The model under review builds one solid part; all positions refer to its coordinate system, in mm. Face numbers are marked on the shaded views. A direction names the side the tool comes from. Coordinates: 2 decimals unless noted, no trailing zeros. Loops run counter-clockwise (first coordinate to the right, second up) from the corner with the lowest first, then second, coordinate; pieces in that order, holes last. Notation, with made-up numbers: M -29.5,-27.75 L -11.5,-27.75 A12 cw -11.5,-18.75 Z; hole C 72.5,40 d7. An arc over 180 degrees is marked long. Use one line per item in the form item = value.
```python
from build123d import *

# Parameters (mm, degrees)
F0_W     = 22
F0_H     = 22
F0_W_2   = 14
F0_H_2   = 14
F1_DEPTH = 1.45
F2_W     = 22
F2_H     = 22
F2_W_2   = 15
F2_H_2   = 15
F3_DEPTH = 7
F4_SIZE  = 3


with BuildPart() as f1:
    # F0 (on Front) → F1 (new body)
    with BuildSketch(Plane.XZ):
        Rectangle(F0_W, F0_H)
        Rectangle(F0_W_2, F0_H_2, mode=Mode.SUBTRACT)
    extrude(amount=F1_DEPTH)

    # F2 (on face) → F3 (join)
    with BuildSketch(Plane.XZ.offset(1.45)):
        Rectangle(F2_W, F2_H)
        Rectangle(F2_W_2, F2_H_2, mode=Mode.SUBTRACT)
    extrude(amount=F3_DEPTH)

    # F4
    f4_edges = [f1.edges().sort_by_distance(p)[0] for p in [
        (-11, -4.225, 11),
        (11, -4.225, 11),
        (11, -4.225, -11),
        (-11, -4.225, -11),
    ]]
    chamfer(f4_edges, length=F4_SIZE)


solid = f1.part
```
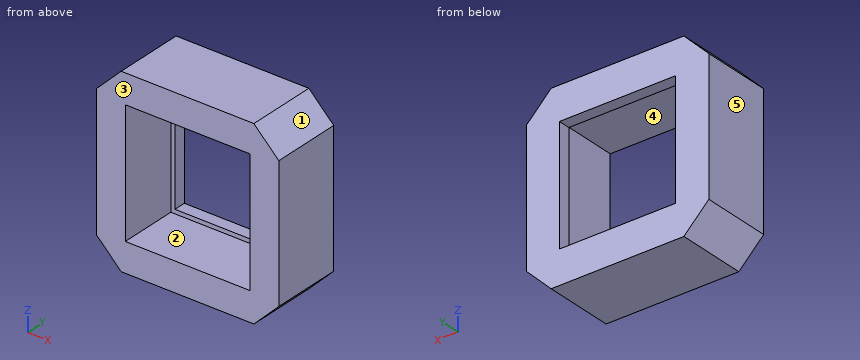
1. Machinability: for the marked faces 4 and 5, which of the approach directions +Z, -Z, +X, -X, +Y, -Y give a long, thin tool a straight path to every point of the face, cutting with its end or side? Answer none if there is none.
Response values:
face_4 = -Y
face_5 = +Z, -Z, -X, +Y, -Y
2. Wall thickness on line 1 along Z through (x, y) = (-6, -4); line 2 along X through (y, z) = (-1, -5.25): over which ranges is each line inside the solid? List them lowest first. Write a range as from..to.
Response values:
line_1 = -11..-7.5, 7.5..11
line_2 = -11..-7, 7..11
3. Add section B-B (z = 6.25). State the section outline as (x, y) points, then the cut area to 3 significant figures.
Response values:
outline = M -11,-8.45 L -7.5,-8.45 L -7.5,-1.45 L -7,-1.45 L -7,0 L -11,0 Z; M 7,-1.45 L 7.5,-1.45 L 7.5,-8.45 L 11,-8.45 L 11,0 L 7,0 Z
area = 60.6 mm^2
4. The part is to be moulded in two halves that separate along X. For the marked faces 1, 2 and 3, say which applies: pulls with the +X half, pulls with the -X half, needs draft (parallel to the pull), parting line crosses it, or undercut.
Response values:
face_1 = pulls with the +X half
face_2 = undercut
face_3 = needs draft
5. Add section A-A (x = 0.5). State the section outline as (y, z) points, then the cut area to 3 significant figures.
Response values:
outline = M -8.45,-11 L 0,-11 L 0,-7 L -1.45,-7 L -1.45,-7.5 L -8.45,-7.5 Z; M -8.45,7.5 L -1.45,7.5 L -1.45,7 L 0,7 L 0,11 L -8.45,11 Z
area = 60.6 mm^2
6. Add section D-D (z = 9.75). State the section outline as (x, y) points, then the cut area to 3 significant figures.
Response values:
outline = M -9.25,-8.45 L 9.25,-8.45 L 9.25,0 L -9.25,0 Z
area = 156 mm^2
7. Add section C-C (y = -2.5). State the section outline as (x, z) points, then the cut area to 3 significant figures.
Response values:
outline = M -11,-8 L -8,-11 L 8,-11 L 11,-8 L 11,8 L 8,11 L -8,11 L -11,8 Z; hole M -7.5,-7.5 L 7.5,-7.5 L 7.5,7.5 L -7.5,7.5 Z
area = 241 mm^2
8. Insertion check: P1, Ø5, axis at x = -4, z = -0.5, coming from the -Y side. The pin has a flat end and moves straight along its axis. Give the tip position at first contact, or say it passes through.
Response values:
P1 = through
